```python
from build123d import *

# Parameters (mm, degrees)
BOSS_EXTRUDE1_DEPTH = 20.6375
BOSS_EXTRUDE2_DEPTH = 20.6375
CUT_EXTRUDE1_DEPTH  = 3.96875
FILLET1_R           = 2.54


with BuildPart() as part:
    # Sketch3 → Boss-Extrude1 (new, symmetric)
    with BuildSketch(Plane(origin=(0, 0, 0), x_dir=(1, 0, 0), z_dir=(0, 1, 0))):
        Polygon((0, 0), (-101.6, 0), (-33.425376719, -47.736385136), align=None)
    extrude(amount=BOSS_EXTRUDE1_DEPTH, both=True)

    # Sketch1 → Boss-Extrude2 (add, symmetric)
    with BuildSketch(Plane(origin=(0, 0, 0), x_dir=(1, 0, 0), z_dir=(0, 1, 0))):
        Polygon((-21.487660076, 10.375160076), (0, 10.375160076), (0, 4.7625), (-15.875, 4.7625), (-15.875, 0), (-39.457964463, 0), align=None)
    extrude(amount=BOSS_EXTRUDE2_DEPTH, both=True)

    # Sketch5 → Cut-Extrude1 (cut, symmetric)
    with BuildSketch(Plane(origin=(0, 0, 0), x_dir=(1, 0, 0), z_dir=(0, 1, 0))):
        Polygon((-56.064295192, 0), (-18.444588457, -26.341602241), (-16.623483272, -23.7407945), (-54.243190006, 2.600807741), align=None)
    extrude(amount=CUT_EXTRUDE1_DEPTH, both=True, mode=Mode.SUBTRACT)

    # Fillet1
    # the kernel refuses this fillet: 2.54 mm, written as the material it adds along each edge
    with BuildSketch(Plane(origin=(-15.875, 20.6375, -4.7625), x_dir=(0, 0, 1), z_dir=(0, -1, 0))) as fillet1_piece_1:
        with BuildLine():
            CenterArc((FILLET1_R, -FILLET1_R), FILLET1_R, 90, 90)
            Line((0, -FILLET1_R), (0, 0))
            Line((0, 0), (FILLET1_R, 0))
        make_face()
    extrude(amount=41.275)
    with BuildSketch(Plane(origin=(-15.875, -20.6375, 0), x_dir=(1, 0, 0), z_dir=(0, 1, 0))) as fillet1_piece_2:
        with BuildLine():
            CenterArc((FILLET1_R, FILLET1_R), FILLET1_R, 180, 90)
            Line((0, FILLET1_R), (0, 0))
            Line((0, 0), (FILLET1_R, 0))
        make_face()
    extrude(amount=41.275)
    with BuildSketch(Plane(origin=(-39.457964463, -20.6375, 0), x_dir=(0.8660254037844413, 0, -0.49999999999999567), z_dir=(0, 1, 0))) as fillet1_piece_3:
        with BuildLine():
            CenterArc((FILLET1_R * 0.267949192431, FILLET1_R), FILLET1_R, 240, 30)
            Line((-FILLET1_R * 0.232050807569, FILLET1_R * 0.133974596216), (0, 0))
            Line((0, 0), (FILLET1_R * 0.267949192431, 0))
        make_face()
    extrude(amount=41.275)
    # the kernel refuses this fillet: 2.54 mm, written as the material it takes off along each edge
    with BuildSketch(Plane(origin=(-56.064295192, 3.96875, 0), x_dir=(-1, 0, 0), z_dir=(0, -1, 0))) as fillet1_2_piece_1:
        with BuildLine():
            CenterArc((FILLET1_R * 0.315298788879, -FILLET1_R), FILLET1_R, 90, 35)
            Line((-FILLET1_R * 0.258277647472, -FILLET1_R * 0.180847955711), (0, 0))
            Line((0, 0), (FILLET1_R * 0.315298788879, 0))
        make_face()
    extrude(amount=7.9375, mode=Mode.SUBTRACT)
    with BuildSketch(Plane(origin=(-50.528851616, 3.96875, 0), x_dir=(1, 0, 0), z_dir=(0, -1, 0))) as fillet1_2_piece_2:
        with BuildLine():
            CenterArc((FILLET1_R * 3.17159480236, FILLET1_R), FILLET1_R, 125, 145)
            Line((FILLET1_R * 2.59801836601, FILLET1_R * 1.81915204429), (0, 0))
            Line((0, 0), (FILLET1_R * 3.17159480236, 0))
        make_face()
    extrude(amount=7.9375, mode=Mode.SUBTRACT)
    with BuildSketch(Plane(origin=(-18.444588457, -3.96875, 26.341602241), x_dir=(-0.5735764363510412, 0, 0.8191520442889952), z_dir=(0, 1, 0))) as fillet1_2_piece_3:
        with BuildLine():
            CenterArc((FILLET1_R, -FILLET1_R), FILLET1_R, 90, 90)
            Line((0, -FILLET1_R), (0, 0))
            Line((0, 0), (FILLET1_R, 0))
        make_face()
    extrude(amount=7.9375, mode=Mode.SUBTRACT)
    with BuildSketch(Plane(origin=(-16.623483272, -3.96875, 23.7407945), x_dir=(0.573576436351041, 0, -0.8191520442889954), z_dir=(0, 1, 0))) as fillet1_2_piece_4:
        with BuildLine():
            CenterArc((FILLET1_R, FILLET1_R), FILLET1_R, 180, 90)
            Line((0, FILLET1_R), (0, 0))
            Line((0, 0), (FILLET1_R, 0))
        make_face()
    extrude(amount=7.9375, mode=Mode.SUBTRACT)
    with BuildSketch(Plane(origin=(0, 32.835736506, 0), x_dir=(-1, 0, 0), z_dir=(0, -1, 0))) as fillet1_2_piece_5:
        with BuildLine():
            CenterArc((FILLET1_R * 1.92098212697, -FILLET1_R), FILLET1_R, 90, 125)
            Line((FILLET1_R * 1.10183008268, -FILLET1_R * 1.57357643635), (0, 0))
            Line((0, 0), (FILLET1_R * 1.92098212697, 0))
        make_face()
    extrude(amount=65.671473013, mode=Mode.SUBTRACT)
    with BuildSketch(Plane(origin=(0, 26.9875, -4.7625), x_dir=(-1, 0, 0), z_dir=(0, -1, 0)), Plane(origin=(0, 26.9875, -10.375160076), x_dir=(0, 0, 1), z_dir=(0, -1, 0))) as fillet1_2_piece_6:
        with BuildLine():
            CenterArc((FILLET1_R, FILLET1_R), FILLET1_R, 180, 90)
            Line((0, FILLET1_R), (0, 0))
            Line((0, 0), (FILLET1_R, 0))
        make_face()
    extrude(amount=53.975, mode=Mode.SUBTRACT)
    with BuildSketch(Plane(origin=(-21.487660076, -22.338977372, -10.375160076), x_dir=(1, 0, 0), z_dir=(0, 1, 0))) as fillet1_2_piece_7:
        with BuildLine():
            CenterArc((FILLET1_R * 0.267949192431, -FILLET1_R), FILLET1_R, 90, 30)
            Line((-FILLET1_R * 0.232050807569, -FILLET1_R * 0.133974596216), (0, 0))
            Line((0, 0), (FILLET1_R * 0.267949192431, 0))
        make_face()
    extrude(amount=44.677954744, mode=Mode.SUBTRACT)
    with BuildSketch(Plane(origin=(-33.425376719, 26.9875, 47.736385136), x_dir=(0.5735764363510407, 0, -0.8191520442889956), z_dir=(0, -1, 0))) as fillet1_2_piece_8:
        with BuildLine():
            CenterArc((FILLET1_R, -FILLET1_R), FILLET1_R, 90, 90)
            Line((0, -FILLET1_R), (0, 0))
            Line((0, 0), (FILLET1_R, 0))
        make_face()
    extrude(amount=53.975, mode=Mode.SUBTRACT)
    with BuildSketch(Plane(origin=(-101.6, -40.777126995, 0), x_dir=(1, 0, 0), z_dir=(0, 1, 0))) as fillet1_2_piece_9:
        with BuildLine():
            CenterArc((FILLET1_R * 3.17159480236, -FILLET1_R), FILLET1_R, 90, 145)
            Line((FILLET1_R * 2.59801836601, -FILLET1_R * 1.81915204429), (0, 0))
            Line((0, 0), (FILLET1_R * 3.17159480236, 0))
        make_face()
    extrude(amount=81.55425399, mode=Mode.SUBTRACT)

    # Sketch7 → Cut-Revolve1 (revolve, cut)
    with BuildSketch(Plane(origin=(-56.865154115, 0, 0), x_dir=(0, 0, -1), z_dir=(1, 0, 0)), mode=Mode.PRIVATE) as cut_revolve1_sk:
        Polygon((0, -18.415), (-1.049252856, -16.66875), (-46.738854795, -16.66875), (-46.738854795, -14.2875), (0, -14.2875), align=None)
    cut_revolve1 = revolve(cut_revolve1_sk.sketch.rotate(Axis((-56.865154115, -14.2875, 46.738854795), (0, 0, -1)), 270), axis=Axis((-56.865154115, -14.2875, 46.738854795), (0, 0, -1)), mode=Mode.SUBTRACT)

    # Mirror1: Cut-Revolve1 across plane
    add(cut_revolve1.mirror(Plane.ZX), mode=Mode.SUBTRACT)


solid = part.part
```
Check sheet for the modelled part. Datum: model origin and axes. Units: mm. A direction names the side the tool comes from. Round coordinates to 2 decimals unless told otherwise and drop trailing zeros. Order: outer loops, then holes, each group sorted by start corner. A loop starts at its lowest first (then second) coordinate and runs counter-clockwise, first axis right, second up. Notation, with made-up numbers: (-10.5, -35) -> (2.5, -35) arc R21 ccw to (2.5, -24) -> close; hole circle Ø5 at (68.25, 61). An arc over 180 degrees is marked (long way). One line per item, written item: value. Start each with the question number.
Q1. Gauge pin test, flat ends, axial feed: pin 1 Ø3 at (x, y) = (-6.5, -0.5) entering from +Z; pin 2 Ø12.5 at (x, y) = (-72, 5) entering from -Z; pin 3 Ø5 at (y, z) = (16.5, 33) entering from -X. Record the tip position at first contact, or that the pin passes through.
Q2. Cross-section at A-A (x = -36.5). Record the boundary of the cut face in (y, z), and give its area (3 significant figures).
Q3. Thickness scan on line 1 (Y direction, x = -46, z = 1.5); line 2 (Y direction, x = -56, z = 11); line 3 (Z direction, x = -12, y = 18). Record the ranges inside material, lowest first.
Q4. Cross-section at C-C (y = -2.5). Record the boundary of the cut face in (x, z) (1 decimal).
Q5. Set-up check for faces 4 (the face through (-33.6, 0.3, 46.7)), 5 (the face through (-8, 0, -4.762)), 6 (the face through (-16.83, -0.06, 22.71)), 7 (the face through (-54.665, -13.375, 17.244)), 8 (the face through (-66, 0, 0)): record each of +Z, -Z, +X, -X, +Y, -Y from which the full face is reachable in a straight line by a thin tool's end or side.
Q6. Mould release check, pull along Y, two halves, no side actions. Record for faces 1 (the face through (-15.09, 0.29, -4.06)), 2 (the face through (-54.665, 13.375, 17.244)), 3 (the face through (-44.91, 0.06, 1.82)): pulls with the +Y half, pulls with the -Y half, needs draft (parallel to the pull), parting line crosses it, or undercut.
Q7. Cross-section at B-B (y = 6.5). Record the boundary of the cut face in (x, z) (1 decimal).
Q8. Cross-section at D-D (z = 18). Record the boundary of the cut face in (x, y), and give its area (3 significant figures).
Completed:
1. pin 1: stops at z = 11.43
1. pin 2: stops at z = 0
1. pin 3: stops at x = -58.04
2. outline: (-20.64, -1.71) -> (20.64, -1.71) -> (20.64, 45.58) -> (-20.64, 45.58) -> close; hole (-3.97, 9.82) -> (3.97, 9.82) -> (3.97, 13.7) -> (-3.97, 13.7) -> close
2. area: 1,920 mm²
3. line 1: y = -20.64 to -3.97, 3.97 to 20.64
3. line 2: y = -20.64 to -16.51, -12.07 to 12.07, 16.51 to 20.64
3. line 3: z = -10.38 to -4.76, 0 to 17.14
4. outline: (-95, 4.6) arc R2.5 ccw to (-93.5, 0) -> (-56.9, 0) arc R2.5 ccw to (-55.4, 0.5) -> (-20.5, 24.9) arc R2.5 ccw to (-19.9, 28.4) -> (-32, 45.7) arc R2.5 ccw to (-35.5, 46.3) -> close; (-43.9, 4.6) arc R2.5 ccw to (-42.5, 0) -> (-40.1, 0) arc R2.5 cw to (-38.9, -0.3) -> (-22.1, -10) arc R2.5 ccw to (-20.8, -10.4) -> (-2.5, -10.4) arc R2.5 ccw to (0, -7.8) -> (0, -7.3) arc R2.5 ccw to (-2.5, -4.8) -> (-13.3, -4.8) arc R2.5 cw to (-15.9, -2.4) arc R2.5 cw to (-13.3, 0) -> (-4.9, 0) arc R2.5 ccw to (-2.8, 4) -> (-15.2, 21.7) arc R2.5 ccw to (-18.7, 22.3) -> close
5. face 4: +Z, +Y, -Y
5. face 5: +X, +Y, -Y
5. face 6: +Z
5. face 7: +Z, -Z
5. face 8: -Z, -X, +Y, -Y
6. face 1: needs draft
6. face 2: undercut
6. face 3: undercut
7. outline: (-95, 4.6) arc R2.5 ccw to (-93.5, 0) -> (-40.1, 0) arc R2.5 cw to (-38.9, -0.3) -> (-22.1, -10) arc R2.5 ccw to (-20.8, -10.4) -> (-2.5, -10.4) arc R2.5 ccw to (0, -7.8) -> (0, -7.3) arc R2.5 ccw to (-2.5, -4.8) -> (-13.3, -4.8) arc R2.5 cw to (-15.9, -2.4) arc R2.5 cw to (-13.3, 0) -> (-4.9, 0) arc R2.5 ccw to (-2.8, 4) -> (-32, 45.7) arc R2.5 ccw to (-35.5, 46.3) -> close
8. outline: (-75.89, -20.64) -> (-12.6, -20.64) -> (-12.6, 20.64) -> (-75.89, 20.64) -> close; hole circle Ø4.76 at (-56.87, -14.29); hole circle Ø4.76 at (-56.87, 14.29); hole (-30.36, -3.97) -> (-24.82, -3.97) -> (-24.82, 3.97) -> (-30.36, 3.97) -> close
8. area: 2,530 mm²
